```python
from build123d import *

# Parameters (mm, degrees)
SKETCH2_W            = 30
SKETCH2_H            = 19.6
SKETCH2_W_2          = 22
SKETCH2_H_2          = 10
BOSS_EXTRUDE2_DEPTH  = 32
SKETCH3_W            = 72
SKETCH3_H            = 50
BOSS_EXTRUDE3_DEPTH  = 6.35
SKETCH4_R            = 1.45
CUT_EXTRUDE1_DEPTH   = 6.35
LPATTERN1_COUNT      = 2
LPATTERN1_PITCH      = 66.000000014
LPATTERN1_COUNT_DIR2 = 2
LPATTERN1_PITCH_DIR2 = 44.000000072
FILLET1_R            = 6.35
FILLET2_R            = 2.54
FILLET3_R            = 2.54


with BuildPart() as part:
    # Sketch2 → Boss-Extrude2 (new body)
    with BuildSketch(Plane(origin=(0, 0, 0), x_dir=(0, 0, -1), z_dir=(1, 0, 0))):
        with Locations((0, -1.55)):
            Rectangle(SKETCH2_W, SKETCH2_H)
        Rectangle(SKETCH2_W_2, SKETCH2_H_2, mode=Mode.SUBTRACT)
    extrude(amount=BOSS_EXTRUDE2_DEPTH)

    # Sketch3 → Boss-Extrude3 (add)
    with BuildSketch(Plane.XZ.offset(11.35)):
        with Locations((16, 0)):
            Rectangle(SKETCH3_W, SKETCH3_H)
    extrude(amount=-BOSS_EXTRUDE3_DEPTH)

    # Sketch4 → Cut-Extrude1 (cut)
    with BuildSketch(Plane(origin=(0, -5, 0), x_dir=(1, 0, 0), z_dir=(0, 1, 0))):
        with Locations(Location((-17, -22.000006, 0), (0, 0, 270))):
            Circle(SKETCH4_R)
    cut_extrude1 = extrude(amount=-CUT_EXTRUDE1_DEPTH, mode=Mode.SUBTRACT)

    # LPattern1: Cut-Extrude1 2 × 2
    with Locations(*[(i * LPATTERN1_PITCH, 0, -j * LPATTERN1_PITCH_DIR2) for i in range(LPATTERN1_COUNT) for j in range(LPATTERN1_COUNT_DIR2) if (i, j) != (0, 0)]):
        add(cut_extrude1, mode=Mode.SUBTRACT)

    # Fillet1
    fillet1_edges = [part.edges().sort_by_distance(p)[0] for p in [
        (0, -5, 13),
        (0, -5, -13),
        (16, -5, 15),
        (32, -5, 13),
        (32, -5, -13),
        (16, -5, -15),
    ]]
    fillet(fillet1_edges, radius=FILLET1_R)

    # Fillet2
    fillet2_edges = [part.edges().sort_by_distance(p)[0] for p in [
        (0, 8.25, 0),
        (16, 8.25, 15),
        (16, 8.25, -15),
        (32, 8.25, 0),
    ]]
    fillet(fillet2_edges, radius=FILLET2_R)

    # Fillet3
    # the kernel refuses this fillet: 2.54 mm, written as the material it takes off along each edge
    with BuildSketch(Plane(origin=(0, 5, -11), x_dir=(0, 1, 0), z_dir=(0, 0, 1))) as fillet3_piece_1:
        with BuildLine():
            CenterArc((FILLET3_R, -FILLET3_R), FILLET3_R, 90, 90)
            Line((0, -FILLET3_R), (0, 0))
            Line((0, 0), (FILLET3_R, 0))
        make_face()
    extrude(amount=22, mode=Mode.SUBTRACT)
    with BuildSketch(Plane(origin=(32, 5, -11), x_dir=(0, 1, 0), z_dir=(0, 0, 1))) as fillet3_piece_2:
        with BuildLine():
            CenterArc((FILLET3_R, FILLET3_R), FILLET3_R, 180, 90)
            Line((0, FILLET3_R), (0, 0))
            Line((0, 0), (FILLET3_R, 0))
        make_face()
    extrude(amount=22, mode=Mode.SUBTRACT)


solid = part.part
```
Design review of the part built by this model. Coordinates are the model's own, in mm. A direction names the side the tool comes from. Coordinates: 2 decimals unless noted, no trailing zeros. Write each loop counter-clockwise with the first axis right and the second up, starting at its lowest first coordinate (ties: lowest second). Pieces come first, ordered by that corner, then holes.
1) Add section D-D (z = -17). Write out the cut boundary in (x, y).
2) To check wall thickness, follow L1, parallel to X at y = -9, z = -22; L2, parallel to Y at x = 28, z = -6.5; L3, parallel to Y at x = 43.5, z = 22.5. State the ranges of each line that lie inside material, in increasing order.
3) Machinability: for faces 4 (the flat face through (32, 4, -13)), 5 (the flat face through (16, 3, -15)), 6 (the cylindrical face through (1.086, 5.457, -0.154)), 7 (the flat face through (16, 8.25, 0)), which of the approach directions +Z, -Z, +X, -X, +Y, -Y give a long, thin tool a straight path to every point of the face, cutting with its end or side? Answer none if there is none.
4) Add section A-A (x = -17). Write out the cut boundary in (y, z), plus the area to 3 significant figures.
5) Insertion check: pin 1 (1.7 mm diameter, centred on x = 49, z = 22, fed in from -Y); pin 2 (2 mm diameter, centred on x = 14, y = 3.5, fed in from +Z); pin 3 (1 mm diameter, centred on x = 5, y = -2, fed in from -Z); pin 4 (4.5 mm diameter, centred on y = 4.5, z = 14, fed in from -X). Each pin has a flat end and moves straight along its axis. Give the tip position at first contact, or say it passes through.
6) Mouldability with a two-part tool opening along X and no side actions: class faces 1 (the cylindrical face through (-16.56, -8.13, 23.38)), 2 (the flat face through (16, 3, 15)), 3 (the flat face through (0, 4, 13)) as +X half, -X half, draft (parallel to the pull), parting line (faces both ways), or undercut.
7) Add section B-B (y = -4). Write out the cut boundary in (x, z), plus the area to 3 significant figures.
8) Add section C-C (x = 6). Write out the cut boundary in (y, z).
Check result:
1. outline: (-20, -11.35) - (52, -11.35) - (52, -5) - (38.35, -5) arc R6.35 cw to (34, -3.28) - (-2, -3.28) arc R6.35 cw to (-6.35, -5) - (-20, -5) - close
2. L1: x = -20 to -18.45, -15.55 to 47.55, 50.45 to 52
2. L2: y = -11.35 to -5, 5 to 8.25
2. L3: y = -11.35 to -5
3. face 4: +Z, -Z, +X, +Y
3. face 5: -Z, +X, -X, +Y
3. face 6: -X
3. face 7: +Z, -Z, +X, -X, +Y
4. outline: (-11.35, -25) - (-5, -25) - (-5, -23.45) - (-11.35, -23.45) - close; (-11.35, -20.55) - (-5, -20.55) - (-5, 20.55) - (-11.35, 20.55) - close; (-11.35, 23.45) - (-5, 23.45) - (-5, 25) - (-11.35, 25) - close
4. area: 281 mm2
5. pin 1: passes through
5. pin 2: stops at z = 15
5. pin 3: stops at z = -16.3
5. pin 4: stops at x = 0
6. face 1: undercut
6. face 2: draft
6. face 3: -X half
7. outline: (-2.93, -17.93) - (34.93, -17.93) - (34.93, -11) - (-2.93, -11) - close; (-2.93, 11) - (34.93, 11) - (34.93, 17.93) - (-2.93, 17.93) - close
7. area: 525 mm2
8. outline: (-11.35, -25) - (-5, -25) - (-5, -21.35) arc R6.35 cw to (1.35, -15) - (5.71, -15) arc R2.54 ccw to (8.25, -12.46) - (8.25, 12.46) arc R2.54 ccw to (5.71, 15) - (1.35, 15) arc R6.35 cw to (-5, 21.35) - (-5, 25) - (-11.35, 25) - close; hole (-5, -11) - (5, -11) - (5, 11) - (-5, 11) - close
